The listing builds one solid part. Answer for the finished solid, in the listing's coordinates (mm). A direction names the side the tool comes from. Coordinates: 2 decimals unless noted, no trailing zeros. Order: outer loops, then holes, each group sorted by start corner. A loop starts at its lowest first (then second) coordinate and runs counter-clockwise, first axis right, second up. Notation, with made-up numbers: (24, 86) -> (71, 86) arc R6 ccw to (71, 91) -> close; hole circle Ø11 at (42, 11). An arc over 180 degrees is marked (long way). Return JSON: item names as keys, results as strings.
Autodesk Fusion 360 part; units mm, degrees
sketch "スケッチ1" plane through (0, 0, 0) normal (0, 0, 1) x (1, 0, 0)
  circle A0 centre (0, 0) radius 25.5
  dimension "d1" = 51
extrude "押し出し1" add sketch "スケッチ1" along normal blind 40
sketch "スケッチ2" plane through (0, 0, 40) normal (0, 0, 1) x (-1, 0, 0)
  circle A0 centre (0, 0) radius 25.5
  circle A1 centre (0, 0) radius 23.5
  dimension "d4" = 47
extrude "押し出し2" cut sketch "スケッチ2" against normal blind 35 contours A1
sketch "スケッチ3" plane through (0, 0, 5) normal (0, 0, 1) x (-1, 0, 0)
  circle A0 centre (0, 0) radius 23.5
  line L0 (7, -7) -> (32, -7)
  line L1 (32, -7) -> (32, -32)
  line L2 (32, -32) -> (7, -32)
  line L3 (7, -32) -> (7, -7)
  line L4 (7, 7) -> (32, 7)
  line L5 (32, 7) -> (32, 32)
  line L6 (32, 32) -> (7, 32)
  line L7 (7, 32) -> (7, 7)
  line L8 (-7, 7) -> (-32, 7)
  line L9 (-32, 7) -> (-32, 32)
  line L10 (-32, 32) -> (-7, 32)
  line L11 (-7, 32) -> (-7, 7)
  line L12 (-7, -7) -> (-32, -7)
  line L13 (-32, -7) -> (-32, -32)
  line L14 (-32, -32) -> (-7, -32)
  line L15 (-7, -32) -> (-7, -7)
  dimension "d7" = 25
  dimension "d8" = 25
  dimension "d9" = 25
  dimension "d10" = 25
  dimension "d11" = 25
  dimension "d12" = 25
  dimension "d13" = 25
  dimension "d14" = 25
extrude "押し出し3" cut sketch "スケッチ3" along normal blind 35 contours A0 L12 L13 L14 L15
extrude "押し出し4" cut sketch "スケッチ3" along normal blind 35 contours A0 L0 L1 L2 L3
extrude "押し出し5" cut sketch "スケッチ3" along normal blind 35 contours A0 L4 L5 L6 L7 | A0 L8 L9 L10 L11
extrude "押し出し6" cut sketch "スケッチ3" against normal blind 5 contours A0 L4 L7 | A0 L0 L3 | A0 L8 L11 | A0 L12 L15
1. The part is cut by section D-D on y = 0. Give the vertices of the cut face in (x, z).
Answer block:
{"outline": "(-25.5, 0) -> (25.5, 0) -> (25.5, 40) -> (23.5, 40) -> (23.5, 5) -> (-23.5, 5) -> (-23.5, 40) -> (-25.5, 40) -> close"}
2. Consider line 1 (Z direction, x = -6.5, y = -21.5); line 2 (Y direction, x = -11.5, z = 3.5); line 3 (Y direction, x = -2.5, z = 26.5). Determine where each line is inside the solid, lowest interval first. Write a range as from..to.
Answer block:
{"line 1": "z = 0..5", "line 2": "y = -22.76..-20.49, -7..7, 20.49..22.76", "line 3": "y = -25.38..-23.37, 23.37..25.38"}
3. The part is cut by section B-B on x = 16. Give the vertices of the cut face in (y, z).
Answer block:
{"outline": "(-19.86, 0) -> (-17.21, 0) -> (-17.21, 5) -> (-19.86, 5) -> close; (-7, 0) -> (7, 0) -> (7, 5) -> (-7, 5) -> close; (17.21, 0) -> (19.86, 0) -> (19.86, 5) -> (17.21, 5) -> close"}
4. Determine the mould class of faces 1 (the face through (23, 7, 22)), 2 (the face through (-7, -23, 22)), 3 (the face through (0, 0, 5)) for opening direction X: pulls with the +X half, pulls with the -X half, needs draft (parallel to the pull), parting line crosses it, or undercut.
Answer block:
{"face 1": "needs draft", "face 2": "pulls with the -X half", "face 3": "undercut"}
5. Each of these flat-tipped pins is pushed along its axis until it touches: pin 1 Ø10 at (x, z) = (9.5, 30.5) entering from +Y; pin 2 Ø4 at (x, z) = (12, 2) entering from +Y; pin 3 Ø4 at (y, z) = (16, 3.5) entering from -X; pin 4 Ø5 at (x, y) = (10, 13) entering from +Z. Where does it stop, or does it pass through?
Answer block:
{"pin 1": "stops at y = 25.1", "pin 2": "stops at y = 23.46", "pin 3": "stops at x = -21.31", "pin 4": "passes through"}
6. The part is cut by section A-A on z = 18.5. Give the vertices of the cut face in (x, y).
Answer block:
{"outline": "(-24.52, -7) -> (-22.43, -7) arc R23.5 cw to (-22.43, 7) -> (-24.52, 7) arc R25.5 ccw to start; (-7, -24.52) arc R25.5 ccw to (7, -24.52) -> (7, -22.43) arc R23.5 cw to (-7, -22.43) -> close; (-7, 22.43) arc R23.5 cw to (7, 22.43) -> (7, 24.52) arc R25.5 ccw to (-7, 24.52) -> close; (22.43, -7) -> (24.52, -7) arc R25.5 ccw to (24.52, 7) -> (22.43, 7) arc R23.5 cw to start"}
7. For faces 4 (the face through (-0.1, -23.5, 22.7)), 5 (the face through (-7, 23, 22)), 6 (the face through (-15, 7, 3)), 7 (the face through (7, 23, 22)), 8 (the face through (0, -24, 40)), determine the directions among +Z, -Z, +X, -X, +Y, -Y from which every point of the face is accessible in a straight line to the end or side of a thin tool.
Answer block:
{"face 4": "+Z", "face 5": "+Z, -X, +Y, -Y", "face 6": "+Z, -Z", "face 7": "+Z, +X, +Y, -Y", "face 8": "+Z, +X, -X, +Y, -Y"}
8. The part is cut by section C-C on y = -12. Give the vertices of the cut face in (x, z).
Answer block:
{"outline": "(-22.5, 0) -> (-20.21, 0) -> (-20.21, 5) -> (-22.5, 5) -> close; (-7, 0) -> (7, 0) -> (7, 5) -> (-7, 5) -> close; (20.21, 0) -> (22.5, 0) -> (22.5, 5) -> (20.21, 5) -> close"}
